from build123d import *

# Parameters (mm, degrees)
EXTRUDE_1_DEPTH = 3.3
SKETCH_2_W      = 57.839960125
SKETCH_2_H      = 3
EXTRUDE_2_DEPTH = 5


with BuildPart() as part:
    # 草图1 → 凸台-拉伸1 (new body)
    with BuildSketch(Plane.XY):
        with BuildLine():
            Line((-49.172249904, -26.54104015), (-49.172249904, -29.54104015))
            Line((-49.172249904, -29.54104015), (33.967710221, -29.54104015))
            ThreePointArc((33.967710221, -29.54104015), (38.626676103, -28.38943192), (42.212581294, -25.199847532))
            ThreePointArc((42.212581294, -25.199847532), (50.170886291, 0.45895985), (42.212581294, 26.117767232))
            ThreePointArc((42.212581294, 26.117767232), (38.626676103, 29.307351619), (33.967710221, 30.45895985))
            Line((33.967710221, 30.45895985), (-49.172249904, 30.45895985))
            Line((-49.172249904, 30.45895985), (-49.172249904, 27.45895985))
            Line((-49.172249904, 27.45895985), (8.667710221, 27.45895985))
            Line((8.667710221, 27.45895985), (8.667710221, 24.420125017))
            Line((8.667710221, 24.420125017), (39.739119972, 24.420125017))
            Line((39.739119972, 24.420125017), (39.739119972, -23.502205318))
            ThreePointArc((39.739119972, -23.502205318), (39.72572916, -23.521645368), (39.712272868, -23.54104015))
            Line((39.712272868, -23.54104015), (8.667710221, -23.54104015))
            Line((8.667710221, -23.54104015), (8.667710221, -26.54104015))
            Line((8.667710221, -26.54104015), (-49.172249904, -26.54104015))
        make_face()
    extrude(amount=EXTRUDE_1_DEPTH)

    # 草图2 → 凸台-拉伸2 (add)
    with BuildSketch(Plane.XY.offset(3.3)):
        with Locations((-20.252269842, -25.04104015)):
            Rectangle(SKETCH_2_W, SKETCH_2_H)
        with BuildLine():
            Line((39.739119972, 24.420125017), (33.967710221, 24.420125017))
            Line((33.967710221, 24.420125017), (33.967710221, -23.54104015))
            Line((33.967710221, -23.54104015), (39.712272868, -23.54104015))
            ThreePointArc((39.712272868, -23.54104015), (39.72572916, -23.521645368), (39.739119972, -23.502205318))
            Line((39.739119972, -23.502205318), (39.739119972, 24.420125017))
        make_face()
        with BuildLine():
            Line((-49.172249904, 30.45895985), (-49.172249904, 27.45895985))
            Line((-49.172249904, 27.45895985), (8.667710221, 27.45895985))
            Line((8.667710221, 27.45895985), (8.667710221, 24.45895985))
            Line((8.667710221, 24.45895985), (33.967710221, 24.45895985))
            Line((33.967710221, 24.45895985), (33.967710221, 24.420125017))
            Line((33.967710221, 24.420125017), (39.739119972, 24.420125017))
            Line((39.739119972, 24.420125017), (39.739119972, -23.502205318))
            ThreePointArc((39.739119972, -23.502205318), (39.72572916, -23.521645368), (39.712272868, -23.54104015))
            Line((39.712272868, -23.54104015), (33.967710221, -23.54104015))
            Line((33.967710221, -23.54104015), (8.667710221, -23.54104015))
            Line((8.667710221, -23.54104015), (8.667710221, -26.54104015))
            Line((8.667710221, -26.54104015), (-49.172249904, -26.54104015))
            Line((-49.172249904, -26.54104015), (-49.172249904, -29.54104015))
            Line((-49.172249904, -29.54104015), (33.967710221, -29.54104015))
            ThreePointArc((33.967710221, -29.54104015), (38.626676103, -28.38943192), (42.212581294, -25.199847532))
            ThreePointArc((42.212581294, -25.199847532), (50.170886291, 0.45895985), (42.212581294, 26.117767232))
            ThreePointArc((42.212581294, 26.117767232), (38.626676103, 29.307351619), (33.967710221, 30.45895985))
            Line((33.967710221, 30.45895985), (-49.172249904, 30.45895985))
        make_face()
        with Locations((-20.252269842, 25.95895985)):
            Rectangle(SKETCH_2_W, SKETCH_2_H)
    extrude(amount=EXTRUDE_2_DEPTH)


solid = part.part
CAD build for the part. Positions are in the model's coordinates, mm. A direction names the side the tool comes from. Give positions to 0.01 mm unless a question says otherwise; leave off trailing zeros. Loops run counter-clockwise (first coordinate to the right, second up) from the corner with the lowest first, then second, coordinate; pieces in that order, holes last. Notation, with made-up numbers: M -39,53.25 L -34,53.25 A5 cw -34,57.25 Z; hole C 78.25,-19 d9. An arc over 180 degrees is marked long. Write each question's results on one line, items separated by ' | '.
Q1. Band-saw the part on D-D on y = -17. Write the cut outline in (x, z), and give its area (3 significant figures).
Geometry check:
outline: M 33.97,3.3 L 39.74,3.3 L 39.74,0 L 46.67,0 L 46.67,8.3 L 33.97,8.3 Z | area: 86.4 mm²
Q2. Band-saw the part on B-B on z = 6. Write the cut outline in (x, y), and give its area (3 significant figures).
Geometry check:
outline: M -49.17,-29.54 L 33.97,-29.54 A10 ccw 42.21,-25.2 A45.34 ccw 42.21,26.12 A10 ccw 33.97,30.46 L -49.17,30.46 L -49.17,24.46 L 33.97,24.46 L 33.97,-23.54 L -49.17,-23.54 Z | area: 1,750 mm²
Q3. Band-saw the part on C-C on x = -15. Write the cut outline in (y, z), and give its area (3 significant figures).
Geometry check:
outline: M -29.54,0 L -26.54,0 L -26.54,3.3 L -23.54,3.3 L -23.54,8.3 L -29.54,8.3 Z; M 24.46,3.3 L 27.46,3.3 L 27.46,0 L 30.46,0 L 30.46,8.3 L 24.46,8.3 Z | area: 79.8 mm²
Q4. Which spindle directions (+Z, -Z, +X, -X, +Y, -Y) get a long thin tool onto all of the face, cutting with end or side? Do faces 1 (the face through (38.687, 29.276, 4.092)), 2 (the face through (-21, 27.459, 2)). Say none if no direction does.
Geometry check:
face 1: +Z, -Z, +X, +Y | face 2: -Z, -X
Q5. Mould opens along Y. For faces 3 (the face through (24, 24.42, 2)), 4 (the face through (-8, -29.541, 4)), 5 (the face through (11, 25, 8.3)), 6 (the face through (50.17, 0.08, 4.09)) say: pulls with the +Y half, pulls with the -Y half, needs draft (parallel to the pull), parting line crosses it, or undercut.
Geometry check:
face 3: undercut | face 4: pulls with the -Y half | face 5: needs draft | face 6: parting line crosses it
Q6. Flat gauge pins, fed straight in: P1, Ø1.5, axis at y = 3.5, z = 4.5, coming from the -X side; P2, Ø2, axis at y = 21, z = 7, coming from the +X side; P3, Ø0.9, axis at x = -17, y = 26, coming from the -Z side; P4, Ø12, axis at x = 33.5, y = 19, coming from the -Z side. Where does each tip first touch, or does it go through?
Geometry check:
P1: stops at x = 33.97 | P2: stops at x = 45.74 | P3: stops at z = 3.3 | P4: stops at z = 0
Q7. Probe probe 1 along Y at (x, z) = (-17.5, 2.75); probe 2 along Y at (x, z) = (-36, 5.75); probe 3 along Z at (x, y) = (-32, -24). List the from-to ranges inside material, lowest first.
Geometry check:
probe 1: y = -29.54 to -26.54, 27.46 to 30.46 | probe 2: y = -29.54 to -23.54, 24.46 to 30.46 | probe 3: z = 3.3 to 8.3
